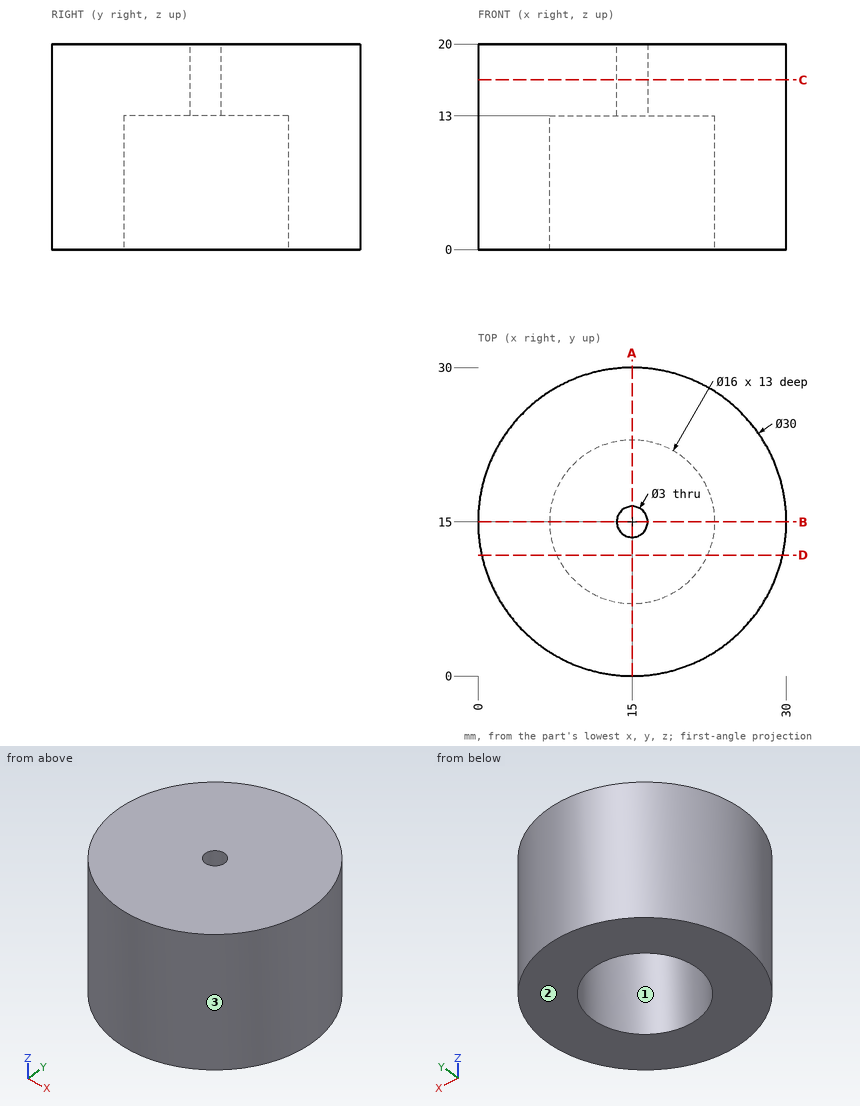
Can you work these out from the drawing? Everything is in mm from the part's minimum corner. Give positions to 0.01 mm unless a question says otherwise; leave off trailing zeros. Loops run counter-clockwise (first coordinate to the right, second up) from the corner with the lowest first, then second, coordinate; pieces in that order, holes last. Notation, with made-up numbers: (79.5, -26.5) - (137.5, -26.5) arc R17 ccw to (137.5, 6.5) - close; hole circle Ø1 at (-22.5, -38.75). An arc over 180 degrees is marked (long way). Answer as a JSON object with one key per item and string values.
Q1. Imagine slicing it at A-A on x = 15. Write out the boundary of the cut face in (y, z), plus the area to 3 significant figures.
Geometry says:
{"outline": "(0, 0) - (7, 0) - (7, 13) - (13.5, 13) - (13.5, 20) - (0, 20) - close; (16.5, 13) - (23, 13) - (23, 0) - (30, 0) - (30, 20) - (16.5, 20) - close", "area": "371 mm²"}
Q2. Imagine slicing it at D-D on y = 11.75. Write out the boundary of the cut face in (x, z).
Geometry says:
{"outline": "(0.36, 0) - (7.69, 0) - (7.69, 13) - (22.31, 13) - (22.31, 0) - (29.64, 0) - (29.64, 20) - (0.36, 20) - close"}
Q3. If I drill on L1, parallel to Y at x = 15, z = 4.75; L2, parallel to Y at x = 15, z = 16.5; L3, parallel to Z at x = 22.25, y = 18.25, over which ranges is the centre line in solid material (lowest first)?
Geometry says:
{"L1": "0 to 7, 23 to 30", "L2": "0 to 13.5, 16.5 to 30", "L3": "13 to 20"}
Q4. If we mould it in two halves opening along Y, with no side actions, what happens to the marked faces 1, 2 and 3? For each: pulls with the +Y half, pulls with the -Y half, needs draft (parallel to the pull), parting line crosses it, or undercut.
Geometry says:
{"face 1": "undercut", "face 2": "needs draft", "face 3": "parting line crosses it"}
Q5. Imagine slicing it at C-C on z = 16.5. Write out the boundary of the cut face in (x, y), plus the area to 3 significant figures.
Geometry says:
{"outline": "circle Ø30 at (15, 15); hole circle Ø3 at (15, 15)", "area": "700 mm²"}
Q6. Will these pins go through, and if not, where does the flat tip stop? P1, Ø3, axis at y = 8.5, z = 13, coming from the +X side; P2, Ø3, axis at x = 21.5, z = 9, coming from the -Y side; P3, Ø8, axis at x = 17.5, y = 11, coming from the -Z side; P4, Ø1, axis at x = 5, z = 16, coming from the +Y side.
Geometry says:
{"P1": "x = 29.14", "P2": "y = 0.86", "P3": "z = 0", "P4": "y = 26.61"}
